```python
from build123d import *

# Parameters (mm, degrees)
SKETCH4_W                    = 20
SKETCH4_H                    = 120
SKETCH4_W_2                  = 120
SKETCH4_H_2                  = 20
SKETCH4_W_3                  = 160
BOSS_EXTRUDE3_DEPTH          = 120
BOSS_EXTRUDE4_DEPTH          = 20
SKETCH21_R                   = 40
CUT_EXTRUDE3_DEPTH           = 25
SKETCH24_W                   = 15
SKETCH24_H                   = 20
SPLIT1_START                 = 97.450277265
SPLIT1_OUTLINE_R             = 45
SPLIT1_OUTLINE_R_2           = 25.75
SPLIT1_DEPTH                 = 42.549722735
SPLIT1_2_DEPTH               = 42.549722735
SPLIT1_3_OUTLINE_R           = 25.75
SPLIT1_3_DEPTH               = 6
SPLIT1_START_2               = 103.450277265
SPLIT1_4_DEPTH               = 8.549722735
SPLIT1_START_3               = 132
SPLIT1_5_DEPTH               = 8
F_5_0_5_DIAMETER_HOLE1_D     = 5
F_5_0_5_DIAMETER_HOLE1_DEPTH = 2.497848452
F_5_0_5_DIAMETER_HOLE1_TIP   = 1.502151548
CUT_EXTRUDE4_DEPTH           = 317.267292017
CUT_EXTRUDE5_DEPTH           = 307.634962129
CUT_EXTRUDE5_DEPTH_BACK      = 307.634962129
FILLET1_R                    = 10


# Read off the part's stored shape, not the designer's step: Split1
with BuildPart() as part:
    # Sketch4 → Boss-Extrude3 (new body)
    with BuildSketch(Plane.XY):
        with Locations((-10, 80)):
            Rectangle(SKETCH4_W, SKETCH4_H)
        with Locations((-60, 10)):
            Rectangle(SKETCH4_W_2, SKETCH4_H_2)
        with Locations((-80, 150)):
            Rectangle(SKETCH4_W_3, SKETCH4_H_2)
    extrude(amount=BOSS_EXTRUDE3_DEPTH)

    # Sketch20 → Boss-Extrude4 (add)
    with BuildSketch(Plane(origin=(0, 160, 0), x_dir=(1, 0, 0), z_dir=(0, 1, 0))):
        with BuildLine():
            Line((-185, -120), (-160, -120))
            Line((-160, -120), (-160, 0))
            Line((-160, 0), (-185, 0))
            ThreePointArc((-185, 0), (-245, -60), (-185, -120))
        make_face()
    extrude(amount=-BOSS_EXTRUDE4_DEPTH)

    # Sketch21 → Cut-Extrude3 (cut)
    with BuildSketch(Plane.XZ.offset(-140)):
        with Locations(Location((-80, 60, 0), (0, 0, 270))):
            Circle(SKETCH21_R)
    extrude(amount=-CUT_EXTRUDE3_DEPTH, mode=Mode.SUBTRACT)

    # Sketch23 → Revolve1 (revolve)
    with BuildSketch(Plane(origin=(0, 0, 60), x_dir=(-1, 0, 0), z_dir=(0, 0, -1)), mode=Mode.PRIVATE) as revolve1_sk:
        Polygon((125, 140), (120, 140), (120, 103.450277265), (105.75, 103.450277265), (105.75, 97.450277265), (125, 97.450277265), align=None)
    revolve(revolve1_sk.sketch.rotate(Axis((-80, 160, 60), (0, -1, 0)), 270), axis=Axis((-80, 160, 60), (0, -1, 0)))

    # Cut-Sweep1: sweep along a path in Sketch25
    with BuildLine(Plane(origin=(0, 132, 0), x_dir=(-1, 0, 0), z_dir=(0, -1, 0))) as cut_sweep1_path:
        Line((125, -80.343984431), (80, -90))
        ThreePointArc((80, -90), (50, -60), (80, -30))
        Line((80, -30), (125, -39.656015569))
    # Sketch24 → Cut-Sweep1 (sweep, cut)
    with BuildSketch(Plane.ZY.offset(125)):
        with Locations((37.5, 122)):
            Rectangle(SKETCH24_W, SKETCH24_H)
    sweep(path=cut_sweep1_path.line, transition=Transition.RIGHT, mode=Mode.SUBTRACT)

    # Split1 outline → Split1 (cut)
    with BuildSketch(Plane(origin=(0, 0, 0), x_dir=(1, 0, 0), z_dir=(0, 1, 0)).offset(SPLIT1_START)):
        with Locations((-80, -60)):
            Circle(SPLIT1_OUTLINE_R)
        with Locations((-80, -60)):
            Circle(SPLIT1_OUTLINE_R_2, mode=Mode.SUBTRACT)
    extrude(amount=SPLIT1_DEPTH, mode=Mode.SUBTRACT)

    # Ø5.0 (5) Diameter Hole1
    with Locations(Plane(origin=(0, 140, 0), x_dir=(-1, 0, 0), z_dir=(0, -1, 0))):
        with Locations((53.75, -14.533666301), (132.5, -60), (53.75, -105.466333699)):
            Hole(F_5_0_5_DIAMETER_HOLE1_D / 2, depth=F_5_0_5_DIAMETER_HOLE1_DEPTH)
            with Locations((0, 0, -(F_5_0_5_DIAMETER_HOLE1_DEPTH + F_5_0_5_DIAMETER_HOLE1_TIP / 2))):  # 118° drill point
                Cone(0, F_5_0_5_DIAMETER_HOLE1_D / 2, F_5_0_5_DIAMETER_HOLE1_TIP, mode=Mode.SUBTRACT)

    # Sketch19 → Cut-Extrude4 (cut, through all)
    with BuildSketch(Plane(origin=(0, 160, 0), x_dir=(1, 0, 0), z_dir=(0, 1, 0))):
        Polygon((-152.526760948, -69.999980109), (-152.526760948, -81), (-212.526760948, -81), (-212.526760948, -39), (-152.526760948, -39), (-152.526760948, -50.000019891), align=None)
    extrude(amount=-CUT_EXTRUDE4_DEPTH, mode=Mode.SUBTRACT)

    # Sketch30 → Cut-Extrude5 (cut, two sides: drawn at the far end of the back side and taken through both)
    with BuildSketch(Plane.XZ.offset(-140).offset(-CUT_EXTRUDE5_DEPTH_BACK)):
        with BuildLine():
            Line((-212.234124069, 23.95), (-142.234124069, 23.95))
            ThreePointArc((-142.234124069, 23.95), (-138.984124069, 20.7), (-142.234124069, 17.45))
            Line((-142.234124069, 17.45), (-212.234124069, 17.45))
            ThreePointArc((-212.234124069, 17.45), (-215.484124069, 20.7), (-212.234124069, 23.95))
        make_face()
        with BuildLine():
            Line((-211.937175822, 102.25), (-141.937175822, 102.25))
            ThreePointArc((-141.937175822, 102.25), (-138.687175822, 99), (-141.937175822, 95.75))
            Line((-141.937175822, 95.75), (-211.937175822, 95.75))
            ThreePointArc((-211.937175822, 95.75), (-215.187175822, 99), (-211.937175822, 102.25))
        make_face()
    extrude(amount=CUT_EXTRUDE5_DEPTH + CUT_EXTRUDE5_DEPTH_BACK, mode=Mode.SUBTRACT)

    # Fillet1
    fillet1_edges = [part.edges().sort_by_distance(p)[0] for p in [
        (0, 160, 60),
    ]]
    fillet(fillet1_edges, radius=FILLET1_R)


with BuildPart() as body_2:
    # Split1 2 outline → Split1 2 (new body)
    with BuildSketch(Plane(origin=(0, 0, 0), x_dir=(1, 0, 0), z_dir=(0, 1, 0)).offset(SPLIT1_START)):
        with BuildLine():
            ThreePointArc((-97.74561888, -24.151806035), (-40, -60), (-97.74561888, -95.848193965))
            Line((-97.74561888, -95.848193965), (-110.465485891, -93.118788767))
            ThreePointArc((-110.465485891, -93.118788767), (-35, -60), (-110.465485891, -26.881211233))
            Line((-110.465485891, -26.881211233), (-97.74561888, -24.151806035))
        make_face()
        with BuildLine():
            ThreePointArc((-116.266630075, -76.873990133), (-120, -60), (-116.266630075, -43.126009867))
            Line((-116.266630075, -43.126009867), (-122.209965285, -44.401319586))
            ThreePointArc((-122.209965285, -44.401319586), (-125, -60), (-122.209965285, -75.598680414))
            Line((-122.209965285, -75.598680414), (-116.266630075, -76.873990133))
        make_face()
    extrude(amount=SPLIT1_2_DEPTH)

    # Split1 3 outline → Split1 3 (add)
    with BuildSketch(Plane(origin=(0, 0, 0), x_dir=(1, 0, 0), z_dir=(0, 1, 0)).offset(SPLIT1_START)):
        with BuildLine():
            ThreePointArc((-97.74561888, -95.848193965), (-40, -60), (-97.74561888, -24.151806035))
            Line((-97.74561888, -24.151806035), (-110.465485891, -26.881211233))
            ThreePointArc((-110.465485891, -26.881211233), (-117.378721889, -34.94344098), (-122.209965285, -44.401319586))
            Line((-122.209965285, -44.401319586), (-116.266630075, -43.126009867))
            ThreePointArc((-116.266630075, -43.126009867), (-120, -60), (-116.266630075, -76.873990133))
            Line((-116.266630075, -76.873990133), (-122.209965285, -75.598680414))
            ThreePointArc((-122.209965285, -75.598680414), (-117.378721889, -85.05655902), (-110.465485891, -93.118788767))
            Line((-110.465485891, -93.118788767), (-97.74561888, -95.848193965))
        make_face()
        with Locations((-80, -60)):
            Circle(SPLIT1_3_OUTLINE_R, mode=Mode.SUBTRACT)
    extrude(amount=SPLIT1_3_DEPTH)

    # Split1 4 outline → Split1 4 (add)
    with BuildSketch(Plane(origin=(0, 0, 0), x_dir=(1, 0, 0), z_dir=(0, 1, 0)).offset(SPLIT1_START_2)):
        with BuildLine():
            ThreePointArc((-116.266630075, -43.126009867), (-108.624043426, -32.059632466), (-97.74561888, -24.151806035))
            Line((-97.74561888, -24.151806035), (-110.465485891, -26.881211233))
            ThreePointArc((-110.465485891, -26.881211233), (-117.378721889, -34.94344098), (-122.209965285, -44.401319586))
            Line((-122.209965285, -44.401319586), (-116.266630075, -43.126009867))
        make_face()
        with BuildLine():
            Line((-110.465485891, -93.118788767), (-97.74561888, -95.848193965))
            ThreePointArc((-97.74561888, -95.848193965), (-108.624043426, -87.940367534), (-116.266630075, -76.873990133))
            Line((-116.266630075, -76.873990133), (-122.209965285, -75.598680414))
            ThreePointArc((-122.209965285, -75.598680414), (-117.378721889, -85.05655902), (-110.465485891, -93.118788767))
        make_face()
    extrude(amount=SPLIT1_4_DEPTH)

    # Split1 5 outline → Split1 5 (add)
    with BuildSketch(Plane(origin=(0, 0, 0), x_dir=(1, 0, 0), z_dir=(0, 1, 0)).offset(SPLIT1_START_3)):
        with BuildLine():
            ThreePointArc((-116.266630075, -43.126009867), (-108.624043426, -32.059632466), (-97.74561888, -24.151806035))
            Line((-97.74561888, -24.151806035), (-110.465485891, -26.881211233))
            ThreePointArc((-110.465485891, -26.881211233), (-117.378721889, -34.94344098), (-122.209965285, -44.401319586))
            Line((-122.209965285, -44.401319586), (-116.266630075, -43.126009867))
        make_face()
        with BuildLine():
            Line((-110.465485891, -93.118788767), (-97.74561888, -95.848193965))
            ThreePointArc((-97.74561888, -95.848193965), (-108.624043426, -87.940367534), (-116.266630075, -76.873990133))
            Line((-116.266630075, -76.873990133), (-122.209965285, -75.598680414))
            ThreePointArc((-122.209965285, -75.598680414), (-117.378721889, -85.05655902), (-110.465485891, -93.118788767))
        make_face()
    extrude(amount=SPLIT1_5_DEPTH)


solid = part.part
```
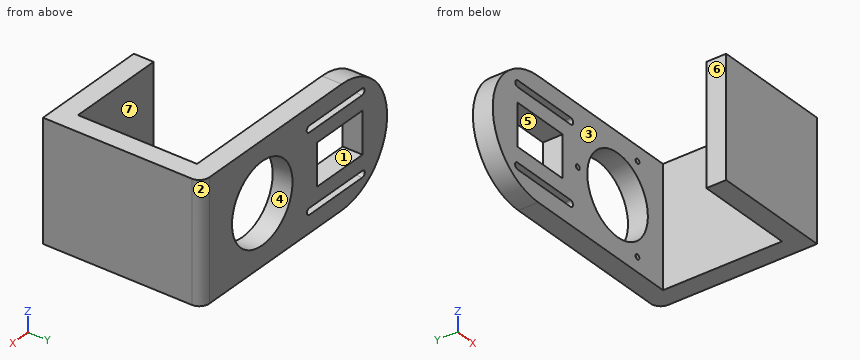
Design review of the part built by this model. Coordinates are the model's own, in mm. Face numbers are marked on the shaded views. A direction names the side the tool comes from. Coordinates: 2 decimals unless noted, no trailing zeros. Loops run counter-clockwise (first coordinate to the right, second up) from the corner with the lowest first, then second, coordinate; pieces in that order, holes last.
Q1. We need section D-D on y = 41. State the section outline as (x, z) points.
Reported:
outline: (-20, 0) - (0, 0) - (0, 120) - (-20, 120) - close
Q2. To check wall thickness, follow line 1 (X direction, y = 144.5, z = 60); line 2 (Y direction, x = -92.5, z = 115); line 3 (Y direction, x = -65, z = 64). State the ranges of each line that lie inside material, in increasing order.
Reported:
line 1: x = -245 to -212.53, -152.53 to -120, -40 to 0
line 2: y = 0 to 20, 140 to 160
line 3: y = 0 to 20
Q3. Tool access review of the marked faces 1, 2, 3 and 4: name each direction out of +Z, -Z, +X, -X, +Y, -Y from which nothing blocks a thin tool from reaching the whole face with its end or side.
Reported:
face 1: +Y, -Y
face 2: +Z, -Z, +X, +Y
face 3: +Z, -Z, -X
face 4: +Y
Q4. We need section C-C on x = -80. State the section outline as (y, z) points.
Reported:
outline: (0, 0) - (20, 0) - (20, 120) - (0, 120) - close; (140, 0) - (160, 0) - (160, 20) - (140, 20) - close; (140, 100) - (160, 100) - (160, 120) - (140, 120) - close
Q5. We need section A-A on x = -146.5. State the section outline as (y, z) points.
Reported:
outline: (140, 0) - (160, 0) - (160, 17.45) - (140, 17.45) - close; (140, 23.95) - (160, 23.95) - (160, 95.75) - (140, 95.75) - close; (140, 102.25) - (160, 102.25) - (160, 120) - (140, 120) - close
Q6. For pin 1 (16 mm diameter, centred on y = 5.5, z = 55.5, fed in from -X); pin 2 (6 mm diameter, centred on x = -132.5, z = 60, fed in from -Y); pin 3 (6 mm diameter, centred on y = 154.5, z = 58.5, fed in from -X); pin 4 (16 mm diameter, centred on x = -187, y = 149, fed in from -Z), all flat-tipped, find the tip position at first contact; note any pin that passes through.
Reported:
pin 1: stops at x = -120
pin 2: stops at y = 140
pin 3: stops at x = -245
pin 4: stops at z = 0
Q7. We need section B-B on z = 49. State the section outline as (x, y) points.
Reported:
outline: (-243.98, 140) - (-212.53, 140) - (-212.53, 160) - (-243.98, 160) - close; (-152.53, 140) - (-118.46, 140) - (-118.46, 160) - (-152.53, 160) - close; (-120, 0) - (0, 0) - (0, 150) arc R10 ccw to (-10, 160) - (-41.54, 160) - (-41.54, 140) - (-20, 140) - (-20, 20) - (-120, 20) - close
Q8. The part is to be moulded in two halves that separate along X. For the marked faces 5, 6 and 7, say which applies: +X half, -X half, draft (parallel to the pull), parting line (faces both ways), or undercut.
Reported:
face 5: undercut
face 6: -X half
face 7: draft
